from build123d import *

# Parameters (mm, degrees)
SKETCH2_W           = 75
SKETCH2_H           = 60
SKETCH2_R           = 7.5
SKETCH2_R_2         = 3.25
SKETCH2_R_3         = 2.5
BOSS_EXTRUDE1_DEPTH = 2


with BuildPart() as part:
    # Sketch2 → Boss-Extrude1 (new body)
    with BuildSketch(Plane.XY):
        with Locations((37.5, 30)):
            Rectangle(SKETCH2_W, SKETCH2_H)
        with Locations((37.5, 45.5)):
            Circle(SKETCH2_R, mode=Mode.SUBTRACT)
        with Locations((64, 12.5)):
            Circle(SKETCH2_R_2, mode=Mode.SUBTRACT)
        with Locations(Location((11, 12.5, 0), (0, 0, 180))):
            Circle(SKETCH2_R_2, mode=Mode.SUBTRACT)
        with Locations((22.5, 45.5)):
            Circle(SKETCH2_R_3, mode=Mode.SUBTRACT)
        with Locations(Location((52.5, 45.5, 0), (0, 0, 180))):
            Circle(SKETCH2_R_3, mode=Mode.SUBTRACT)
    extrude(amount=BOSS_EXTRUDE1_DEPTH)


solid = part.part
The listing builds one solid part. Answer for the finished solid, in the listing's coordinates (mm). Coordinates: 2 decimals unless noted, no trailing zeros. Write each loop counter-clockwise with the first axis right and the second up, starting at its lowest first coordinate (ties: lowest second). Pieces come first, ordered by that corner, then holes. Notation, with made-up numbers: M 1,4.25 L 52,4.25 A7 cw 52,8.25 Z; hole C 48.5,58.5 d10. An arc over 180 degrees is marked long. Write each question's results on one line, items separated by ' | '.
Item 1: For a pull along Y with two mould halves and no side action, classify faces 1 (the face through (37, 60, 1)), 2 (the face through (50.19, 46.46, 0.99)), 3 (the face through (37, 30, 0)) as released by +Y, released by -Y, zero draft, split by the parting line, or undercut.
Answer below:
face 1: released by +Y | face 2: undercut | face 3: zero draft
Item 2: Consider probe 1 along Y at (x, z) = (52.5, 1.3); probe 2 along Y at (x, z) = (64, 0.4); probe 3 along X at (y, z) = (14, 1.75). Determine where each line is inside the solid, lowest interval first. Write a range as [from, to].
Answer below:
probe 1: [0, 43], [48, 60] | probe 2: [0, 9.25], [15.75, 60] | probe 3: [0, 8.12], [13.88, 61.12], [66.88, 75]
Item 3: The part is cut by section B-B on x = 11. Determine the outline of the cut face in (y, z).
Answer below:
outline: M 0,0 L 9.25,0 L 9.25,2 L 0,2 Z; M 15.75,0 L 60,0 L 60,2 L 15.75,2 Z
Item 4: The part is cut by section A-A on y = 45.5. Determine the outline of the cut face in (x, z).
Answer below:
outline: M 0,0 L 20,0 L 20,2 L 0,2 Z; M 25,0 L 30,0 L 30,2 L 25,2 Z; M 45,0 L 50,0 L 50,2 L 45,2 Z; M 55,0 L 75,0 L 75,2 L 55,2 Z
Item 5: The part is cut by section C-C on y = 12.5. Determine the outline of the cut face in (x, z), and give its area (3 significant figures).
Answer below:
outline: M 0,0 L 7.75,0 L 7.75,2 L 0,2 Z; M 14.25,0 L 60.75,0 L 60.75,2 L 14.25,2 Z; M 67.25,0 L 75,0 L 75,2 L 67.25,2 Z | area: 124 mm2
Item 6: The part is cut by section D-D on z = 1.2. Determine the outline of the cut face in (x, y).
Answer below:
outline: M 0,0 L 75,0 L 75,60 L 0,60 Z; hole C 11,12.5 d6.5; hole C 22.5,45.5 d5; hole C 37.5,45.5 d15; hole C 52.5,45.5 d5; hole C 64,12.5 d6.5
